from build123d import *

# Parameters (mm, degrees)
BOSS_EXTRU_1_DEPTH = 3
COQUE1_T           = 1.5


with BuildPart() as part:
    # Esquisse1 → Boss.-Extru.1 (new body)
    with BuildSketch(Plane.XY):
        with BuildLine():
            Line((-24.48, -10.5), (24.48, -10.5))
            ThreePointArc((24.48, -10.5), (25.378025612, -10.128025612), (25.75, -9.23))
            Line((25.75, -9.23), (25.75, 9.23))
            ThreePointArc((25.75, 9.23), (25.378025612, 10.128025612), (24.48, 10.5))
            Line((24.48, 10.5), (-24.48, 10.5))
            ThreePointArc((-24.48, 10.5), (-25.378025612, 10.128025612), (-25.75, 9.23))
            Line((-25.75, 9.23), (-25.75, -9.23))
            ThreePointArc((-25.75, -9.23), (-25.378025612, -10.128025612), (-24.48, -10.5))
        make_face()
    extrude(amount=BOSS_EXTRU_1_DEPTH)

    # Coque1
    coque1_openings = [part.faces().sort_by_distance(p)[0] for p in [
        (0, 0, 3),
    ]]
    offset(amount=COQUE1_T, openings=coque1_openings, kind=Kind.INTERSECTION)


solid = part.part
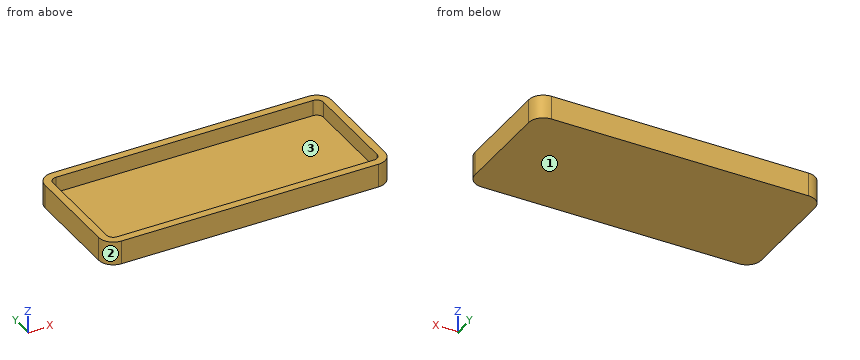
For this review, take the finished solid that the model builds, in its own axes (mm). Face numbers are marked on the shaded views. Round coordinates to 2 decimals unless told otherwise and drop trailing zeros. Write each loop counter-clockwise with the first axis right and the second up, starting at its lowest first coordinate (ties: lowest second). Pieces come first, ordered by that corner, then holes. Notation, with made-up numbers: (-15.5, 4) -> (7.5, 4) arc R24 ccw to (7.5, 19) -> close; hole circle Ø2 at (87.5, 8). An arc over 180 degrees is marked (long way). Use CSV: the item, a comma, the result in double quotes.
(1) Clearance check with a flat-ended pin moving along its axis: P1, Ø8, axis at x = 10.5, y = -2, coming from the +Z side. State where the tip first meets the part, or that it passes through.
Computed values:
P1,"z = 0"
(2) Consider section A-A, the plane x = -19. Give the boundary of the cut face in (y, z).
Computed values:
outline,"(-12, -1.5) -> (12, -1.5) -> (12, 3) -> (10.5, 3) -> (10.5, 0) -> (-10.5, 0) -> (-10.5, 3) -> (-12, 3) -> close"
(3) To check wall thickness, follow L1, parallel to Y at x = -7.5, z = 1.8; L2, parallel to X at y = 7.5, z = 0.5; L3, parallel to Z at x = 0, y = -0.25. State the ranges of each line that lie inside material, in increasing order. Write a range as [from, to].
Computed values:
L1,"[-12, -10.5], [10.5, 12]"
L2,"[-27.25, -25.75], [25.75, 27.25]"
L3,"[-1.5, 0]"
(4) Consider section B-B, the plane z = 0.9. Give the boundary of the cut face in (x, y), plus the area to 3 significant figures.
Computed values:
outline,"(-27.25, -9.23) arc R2.77 ccw to (-24.48, -12) -> (24.48, -12) arc R2.77 ccw to (27.25, -9.23) -> (27.25, 9.23) arc R2.77 ccw to (24.48, 12) -> (-24.48, 12) arc R2.77 ccw to (-27.25, 9.23) -> close; hole (-25.75, -9.23) arc R1.27 ccw to (-24.48, -10.5) -> (24.48, -10.5) arc R1.27 ccw to (25.75, -9.23) -> (25.75, 9.23) arc R1.27 ccw to (24.48, 10.5) -> (-24.48, 10.5) arc R1.27 ccw to (-25.75, 9.23) -> close"
area,"221 mm²"
(5) Consider section C-C, the plane y = 5. Give the boundary of the cut face in (x, z).
Computed values:
outline,"(-27.25, -1.5) -> (27.25, -1.5) -> (27.25, 3) -> (25.75, 3) -> (25.75, 0) -> (-25.75, 0) -> (-25.75, 3) -> (-27.25, 3) -> close"
(6) Draft analysis for pull direction X (two halves, no side actions). For the marked faces 1, 2 and 3, state which applies: +X half, -X half, draft (parallel to the pull), parting line (faces both ways), or undercut.
Computed values:
face 1,"draft"
face 2,"-X half"
face 3,"undercut"
